Design review of the part built by this model. Coordinates are the model's own, in mm. Face numbers are marked on the shaded views. A direction names the side the tool comes from. Give positions to 0.01 mm unless a question says otherwise; leave off trailing zeros. Order: outer loops, then holes, each group sorted by start corner. A loop starts at its lowest first (then second) coordinate and runs counter-clockwise, first axis right, second up.
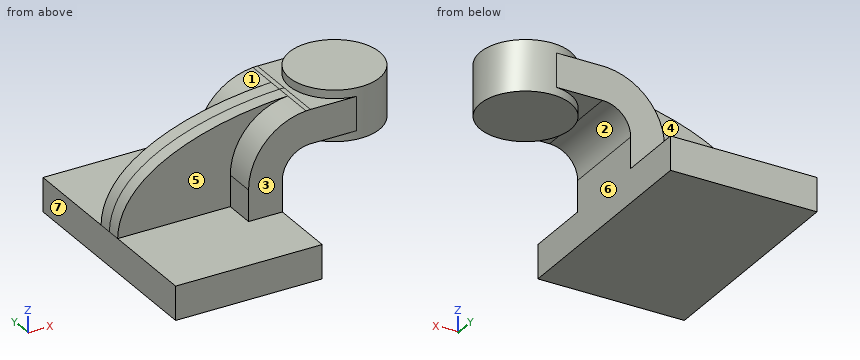
```python
from build123d import *

# Parameters (mm, degrees)
F1_DEPTH = 63.5
F0_W     = 25.2717524765
F0_H     = 19.05
F2_DEPTH = 25.4
F3_DEPTH = 7.9375


with BuildPart() as f1:
    # F0 (on Front) → F1 (new body, symmetric)
    with BuildSketch(Plane.XZ):
        Polygon((22.225, 9.525), (-41.275, 9.525), (-41.275, -9.525), (41.275, -9.525), (41.275, 9.525), align=None)
    extrude(amount=F1_DEPTH, both=True)

    # F0 (on Front) → F2 (join, symmetric)
    with BuildSketch(Plane.XZ):
        with BuildLine():
            Line((22.225, 27.0002), (22.225, 9.525))
            Line((22.225, 9.525), (41.275, 9.525))
            Line((41.275, 9.525), (41.275, 27.0002))
            ThreePointArc((41.275, 27.0002), (45.9246798487, 38.2255201513), (57.15, 42.8752))
            Line((57.15, 42.8752), (60.325, 42.8752))
            Line((60.325, 42.8752), (60.325, 61.9252))
            Line((60.325, 61.9252), (57.15, 61.9252))
            add(Edge.make_bspline(
                [(54.6000717025, 61.8319885082), (55.4560192886, 61.8684142099), (56.3061980805, 61.8994538624), (57.15, 61.9252)],
                knots=[109.2208050055, 109.2208050055, 109.2208050055, 109.2208050055, 111.5045361635, 111.5045361635, 111.5045361635, 111.5045361635], degree=3))
            ThreePointArc((54.6000717025, 61.8319885082), (31.5686408611, 50.7772832863), (22.225, 27.0002))
        make_face()
        with Locations((72.9608762383, 52.4002)):
            Rectangle(F0_W, F0_H)
    extrude(amount=F2_DEPTH, both=True)

    # F0 (on Front) → F3 (join, symmetric)
    with BuildSketch(Plane.XZ):
        with BuildLine():
            add(Edge.make_bspline(
                [(-41.275, 9.525), (-40.467228221, 46.0283825341), (13.6638677739, 60.0899075916), (54.6000717025, 61.8319885082)],
                knots=[0, 0, 0, 0, 109.2208050055, 109.2208050055, 109.2208050055, 109.2208050055], degree=3))
            Line((-41.275, 9.525), (22.225, 9.525))
            Line((22.225, 9.525), (22.225, 27.0002))
            ThreePointArc((22.225, 27.0002), (31.5686408611, 50.7772832863), (54.6000717025, 61.8319885082))
        make_face()
    extrude(amount=F3_DEPTH, both=True)

    # F0 (on Front) → F4 (revolve)
    with BuildSketch(Plane.XZ):
        Polygon((85.5967524765, 66.675), (85.5967524765, 61.9252), (85.5967524765, 42.8752), (85.5967524765, 38.1), (111.125, 38.1), (111.125, 66.675), align=None)
    revolve(axis=Axis((85.5967524765, 0, 52.3875), (0, 0, 1)))


solid = f1.part
```
1. For pin 1 (19 mm diameter, centred on y = -13, z = 20, fed in from -X); pin 2 (2 mm diameter, centred on x = 20, y = 13, fed in from +Z) (3 decimals); pin 3 (4 mm diameter, centred on y = -7, z = 43.5, fed in from -X), all flat-tipped, find the tip position at first contact; note any pin that passes through.
Recorded:
pin 1: stops at x = -41.14
pin 2: stops at z = 9.525
pin 3: stops at x = -21.61
2. Machinability: for the marked faces 4, 5, 6 and 7, which of the approach directions +Z, -Z, +X, -X, +Y, -Y give a long, thin tool a straight path to every point of the face, cutting with its end or side? Answer none if there is none.
Recorded:
face 4: +Z, -X, +Y
face 5: +Z, -X, -Y
face 6: -Z, +X, +Y, -Y
face 7: +Z, -Z, -X, +Y, -Y
3. Draft analysis for pull direction X (two halves, no side actions). For the marked faces 1, 2 and 3, state which applies: pulls with the +X half, pulls with the -X half, needs draft (parallel to the pull), parting line crosses it, or undercut.
Recorded:
face 1: pulls with the -X half
face 2: undercut
face 3: needs draft
4. Take a section at A-A (x = 65). State the section outline as (y, z) points (3 decimals).
Recorded:
outline: (-25.4, 42.875) - (-15.082, 42.875) - (-15.082, 38.1) - (15.082, 38.1) - (15.082, 42.875) - (25.4, 42.875) - (25.4, 61.925) - (15.082, 61.925) - (15.082, 66.675) - (-15.082, 66.675) - (-15.082, 61.925) - (-25.4, 61.925) - close
5. Take a section at B-B (y = 30). State the section outline as (x, z) points (3 decimals).
Recorded:
outline: (-41.275, -9.525) - (41.275, -9.525) - (41.275, 9.525) - (-41.275, 9.525) - close
6. For line 1 along Z through (x, y) = (31, 54) (3 decimals); line 2 along Y through (x, z) = (54, 53); line 3 along X through (y, z) = (-9, 16) (3 decimals), list the stretches that pass through material, from the lowest coordinate up.
Recorded:
line 1: z = -9.525 to 9.525
line 2: y = -25.4 to 25.4
line 3: x = 22.225 to 41.275
